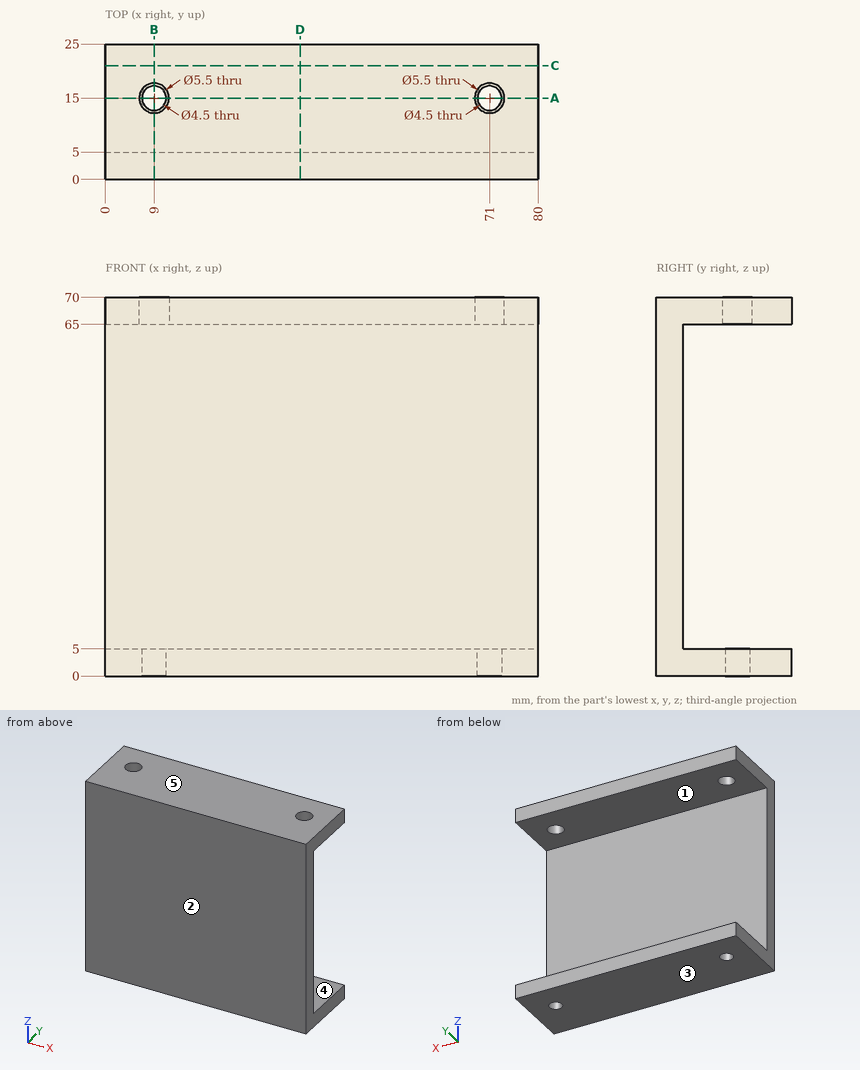
Can you work these out from the drawing? Everything is in mm from the part's minimum corner. A direction names the side the tool comes from. Coordinates: 2 decimals unless noted, no trailing zeros. Write each loop counter-clockwise with the first axis right and the second up, starting at its lowest first coordinate (ties: lowest second). Pieces come first, ordered by that corner, then holes. Notation, with made-up numbers: (-25, 47.25) -> (17, 47.25) arc R21 ccw to (17, 66.25) -> close; hole circle Ø2 at (0, 12.25). An arc over 180 degrees is marked (long way). Return JSON: item names as keys, results as strings.
(1) Imagine slicing it at C-C, the plane y = 21. Please give me the cut outline in (x, z), then the cut area to 3 significant figures.
Numbers:
{"outline": "(0, 0) -> (80, 0) -> (80, 5) -> (0, 5) -> close; (0, 65) -> (80, 65) -> (80, 70) -> (0, 70) -> close", "area": "800 mm2"}
(2) Imagine slicing it at B-B, the plane x = 9. Please give me the cut outline in (y, z).
Numbers:
{"outline": "(0, 0) -> (12.75, 0) -> (12.75, 5) -> (5, 5) -> (5, 65) -> (12.25, 65) -> (12.25, 70) -> (0, 70) -> close; (17.25, 0) -> (25, 0) -> (25, 5) -> (17.25, 5) -> close; (17.75, 65) -> (25, 65) -> (25, 70) -> (17.75, 70) -> close"}
(3) Imagine slicing it at A-A, the plane y = 15. Please give me the cut outline in (x, z), then the cut area to 3 significant figures.
Numbers:
{"outline": "(0, 0) -> (6.75, 0) -> (6.75, 5) -> (0, 5) -> close; (0, 65) -> (6.25, 65) -> (6.25, 70) -> (0, 70) -> close; (11.25, 0) -> (68.75, 0) -> (68.75, 5) -> (11.25, 5) -> close; (11.75, 65) -> (68.25, 65) -> (68.25, 70) -> (11.75, 70) -> close; (73.25, 0) -> (80, 0) -> (80, 5) -> (73.25, 5) -> close; (73.75, 65) -> (80, 65) -> (80, 70) -> (73.75, 70) -> close", "area": "700 mm2"}
(4) Imagine slicing it at D-D, the plane x = 36. Please give me the cut outline in (y, z), then the cut area to 3 significant figures.
Numbers:
{"outline": "(0, 0) -> (25, 0) -> (25, 5) -> (5, 5) -> (5, 65) -> (25, 65) -> (25, 70) -> (0, 70) -> close", "area": "550 mm2"}
(5) I need wall thicknesses on L1, parallel to Z at x = 57, y = 23.5; L2, parallel to Y at x = 9, z = 68.85; L3, parallel to Y at x = 51, z = 31. Which ranges of each line are inside material? Lowest first, please.
Numbers:
{"L1": "z = 0 to 5, 65 to 70", "L2": "y = 0 to 12.25, 17.75 to 25", "L3": "y = 0 to 5"}
(6) Which directions (+Z, -Z, +X, -X, +Y, -Y) give clear straight access to the entire face, cutting with the end or side of a thin tool? Please do the marked faces 1 and 2.
Numbers:
{"face 1": "+X, -X, +Y", "face 2": "+Z, -Z, +X, -X, -Y"}
(7) We'd pull the mould along Z, two halves only. Please class the marked faces 3, 4 and 5: +Z half, -Z half, draft (parallel to the pull), parting line (faces both ways), or undercut.
Numbers:
{"face 3": "-Z half", "face 4": "undercut", "face 5": "+Z half"}
(8) I'm going to push flat-ended pins straight in: pin 1 (2 mm diameter, centred on x = 27, z = 42.5, fed in from +Y); pin 2 (5 mm diameter, centred on x = 71, y = 15, fed in from +Z); pin 3 (3.5 mm diameter, centred on x = 9, y = 15, fed in from +Z). Where does each tip first touch, or does it pass through?
Numbers:
{"pin 1": "stops at y = 5", "pin 2": "stops at z = 5", "pin 3": "passes through"}
